Design review of the part built by this model. Coordinates are the model's own, in mm. Face numbers are marked on the shaded views. A direction names the side the tool comes from. Round coordinates to 2 decimals unless told otherwise and drop trailing zeros. Write each loop counter-clockwise with the first axis right and the second up, starting at its lowest first coordinate (ties: lowest second). Pieces come first, ordered by that corner, then holes.
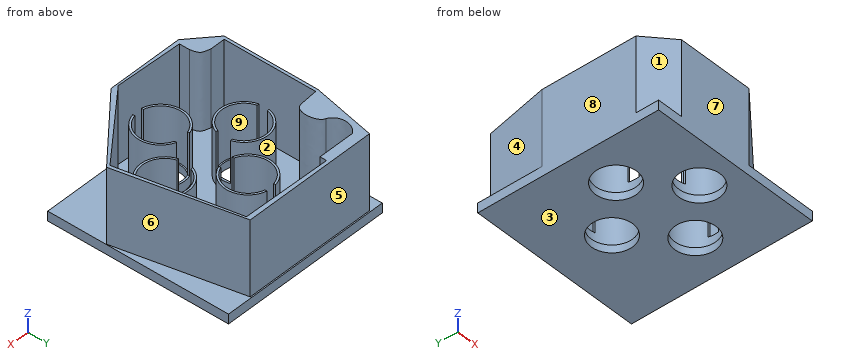
from build123d import *

# Parameters (mm, degrees)
F1_DEPTH  = 220
F3_W      = 450
F3_H      = 470
F4_DEPTH  = 25
F5_DEPTH  = 200
F6_R      = 53.5
F7_DEPTH  = 20
F6_R_2    = 62
F6_R_3    = 57
F8_DEPTH  = 154
F9_W      = 25.5
F9_H      = 90.3576454148
F9_W_2    = 90.3576454148
F9_H_2    = 25.5
F10_DEPTH = 175


with BuildPart() as f1:
    # F0 (on Top) → F1 (new body)
    with BuildSketch(Plane.XY):
        Polygon((-204.7800719738, 171.1511015892), (-238.562181592, 7.3397289511), (-238.562181592, -236.6909831762), (-171.305090189, -295.6561148167), (26.1666476727, -295.6561148167), (210.4326635599, -143.6366438866), (144.4040089846, 171.1511015892), align=None)
    extrude(amount=F1_DEPTH)

    # F3 (on Top) → F4 (join)
    with BuildSketch(Plane.XY):
        with Locations((-13.562181592, -60.6561148167)):
            Rectangle(F3_W, F3_H)
    extrude(amount=F4_DEPTH)

    # F2 (on face) → F5 (cut)
    with BuildSketch(Plane.XY.offset(220)):
        with BuildLine():
            Line((141.9471204281, 159.1738164425), (-88.6924937367, 162.5520288944))
            Line((-88.6924937367, 162.5520288944), (-88.6924937367, 145.6609666348))
            Line((-88.6924937367, 145.6609666348), (-182.9752624035, 145.6609666348))
            add(Edge.make_bspline(
                [(-182.9752624035, 145.6609666348), (-207.5440585613, 131.841018796), (-210.6151580811, 91.9167175889), (-182.9752624035, 77.1754458547)],
                knots=[0, 0, 0, 0, 68.4855207801, 68.4855207801, 68.4855207801, 68.4855207801], degree=3))
            add(Edge.make_bspline(
                [(-182.9752624035, 77.1754458547), (-164.8557782173, 75.025677681), (-155.0282537937, 17.2889921814), (-182.9752624035, 12.0681189001)],
                knots=[0, 0, 0, 0, 65.1073269546, 65.1073269546, 65.1073269546, 65.1073269546], degree=3))
            Line((-182.9752624035, 12.0681189001), (-231.1915457249, 7.7685844153))
            Line((-231.1915457249, 7.7685844153), (-231.1915457249, -229.9345582724))
            Line((-231.1915457249, -229.9345582724), (-191.8814480305, -229.9345582724))
            add(Edge.make_bspline(
                [(-191.8814480305, -229.9345582724), (-168.2339906693, -236.6909831762), (-168.2339906693, -236.6909831762), (-163.0131155252, -259.417116642)],
                knots=[0, 0, 0, 0, 41.2625964967, 41.2625964967, 41.2625964967, 41.2625964967], degree=3))
            Line((-163.0131155252, -259.417116642), (-163.0131155252, -285.8285903931))
            Line((-163.0131155252, -285.8285903931), (10.1969307289, -291.0494506359))
            Line((10.1969307289, -291.0494506359), (201.833575964, -142.4082070589))
            Line((201.833575964, -142.4082070589), (141.9471204281, 159.1738164425))
        make_face()
    extrude(amount=-F5_DEPTH, mode=Mode.SUBTRACT)

    # F6 (on Top) → F7 (cut, through all)
    with BuildSketch(Plane.XY):
        with Locations((-14.6330455318, 24.2691934109)):
            Circle(F6_R)
        with Locations((-128.4027075395, -87.3125935497)):
            Circle(F6_R)
        with Locations((-14.7721923306, -203.1711548904)):
            Circle(F6_R)
        with Locations((98.9974696771, -91.5893679298)):
            Circle(F6_R)
    extrude(amount=F7_DEPTH, mode=Mode.SUBTRACT)

    # F6 (on Top) → F8 (join)
    with BuildSketch(Plane.XY):
        with Locations((98.9974696771, -91.5893679298)):
            Circle(F6_R_2)
        with Locations((98.9974696771, -91.5893679298)):
            Circle(F6_R_3, mode=Mode.SUBTRACT)
        with Locations((-14.6330455318, 24.2691934109)):
            Circle(F6_R_2)
        with Locations((-14.6330455318, 24.2691934109)):
            Circle(F6_R_3, mode=Mode.SUBTRACT)
        with Locations((-128.4027075395, -87.3125935497)):
            Circle(F6_R_2)
        with Locations((-128.4027075395, -87.3125935497)):
            Circle(F6_R_3, mode=Mode.SUBTRACT)
        with Locations((-14.7721923306, -203.1711548904)):
            Circle(F6_R_2)
        with Locations((-14.7721923306, -203.1711548904)):
            Circle(F6_R_3, mode=Mode.SUBTRACT)
    extrude(amount=F8_DEPTH)

    # F9 (on face) → F10 (cut)
    with BuildSketch(Plane.XY.offset(220)):
        Polygon((-14.3728665248, -89.0469396694), (4.8721171106, -89.0469396694), (4.8821498398, -89.0469396694), (4.8821498398, -69.801956034), (-14.3728665248, -69.801956034), align=None)
        Polygon((4.8721171106, -108.301956034), (4.8721171106, -89.0469396694), (-14.3728665248, -89.0469396694), (-14.3728665248, -108.2919233048), (-14.3728665248, -108.301956034), align=None)
        Polygon((4.8821498398, -89.0469396694), (4.8721171106, -89.0469396694), (4.8721171106, -108.301956034), (89.2823901994, -108.301956034), (89.2823901994, -101.801956034), (89.2823901994, -76.301956034), (89.2823901994, -69.801956034), (4.8821498398, -69.801956034), align=None)
        Polygon((-14.3728665248, -108.2919233048), (-14.3728665248, -89.0469396694), (-33.6178501602, -89.0469396694), (-33.6278828894, -89.0469396694), (-33.6278828894, -108.2919233048), align=None)
        Polygon((-33.6178501602, -89.0469396694), (-14.3728665248, -89.0469396694), (-14.3728665248, -69.801956034), (-14.3728665248, -69.7919233048), (-33.6178501602, -69.7919233048), align=None)
        Polygon((4.8721171106, -192.7021963936), (4.8721171106, -108.301956034), (-14.3728665248, -108.301956034), (-14.3728665248, -108.2919233048), (-33.6278828894, -108.2919233048), (-33.6278828894, -192.7021963936), (-27.1278828894, -192.7021963936), (-1.6278828894, -192.7021963936), align=None)
        Polygon((-14.3728665248, -69.801956034), (4.8821498398, -69.801956034), (4.8821498398, 14.6083170548), (-1.6178501602, 14.6083170548), (-27.1178501602, 14.6083170548), (-33.6178501602, 14.6083170548), (-33.6178501602, -69.7919233048), (-14.3728665248, -69.7919233048), align=None)
        Polygon((-33.6278828894, -89.0469396694), (-33.6178501602, -89.0469396694), (-33.6178501602, -69.7919233048), (-118.028123249, -69.7919233048), (-118.028123249, -76.2919233048), (-118.028123249, -101.7919233048), (-118.028123249, -108.2919233048), (-33.6278828894, -108.2919233048), align=None)
        with Locations((-14.3778828894, -237.881019101)):
            Rectangle(F9_W, F9_H)
        with Locations((134.4612129068, -89.051956034)):
            Rectangle(F9_W_2, F9_H_2)
        with Locations((-14.3678501602, 59.7871397622)):
            Rectangle(F9_W, F9_H)
        with Locations((-163.2069459564, -89.0419233048)):
            Rectangle(F9_W_2, F9_H_2)
    extrude(amount=-F10_DEPTH, mode=Mode.SUBTRACT)


solid = f1.part
1) For line 1 along X through (y, z) = (-125.5, 57.5); line 2 along X through (y, z) = (30.5, 88.5); line 3 along Y through (x, z) = (-60, 138), list the stretches that pass through material, from the lowest coordinate up.
2) The part is to be moulded in two halves that separate along X. For the marked faces 6, 7, 8 and 9, say which applies: pulls with the +X half, pulls with the -X half, needs draft (parallel to the pull), parting line crosses it, or undercut.
3) Add section A-A on x = -10. Count the separate pieces of the cut face and the enclosed holes in it, and give its area (3 significant figures).
4) For P1, Ø4, axis at x = -9.5, y = -144, coming from the +Z side; P2, Ø2.5, axis at x = 41.5, z = 89, coming from the +Y side; P3, Ø4, axis at x = 76.5, z = 97.5, coming from the -Y side; P4, Ø6, axis at y = -163, z = 26, coming from the +X side, all flat-tipped, find the tip position at first contact; note any pin that passes through.
5) For the marked faces 1, 2, 3, 4 and 5, list the 3-axis set-ups (+Z, -Z, +X, -X, +Y, -Y) from which the entire face can be reached by the end or side of a thin tool; tool diameter is ignored.
6) Add section D-D on y = -10.5. State the section outline as (x, z) points, and give its area (3 significant figures).
7) Add section C-C on x = 110.5. State the section outline as (y, z) points, and give its area (3 significant figures).
Computed:
1. line 1: x = -238.56 to -231.19, -177.25 to -170.72, -86.09 to -79.56, 47.09 to 53.18, 144.81 to 150.9, 198.48 to 206.63
1. line 2: x = -233.79 to -166.59, -76.32 to -71.29, 42.03 to 47.05, 167.5 to 173.91
1. line 3: y = -295.66 to -288.93, -245.58 to -237.86, -168.48 to -160.76, -17.99 to -10.24, 58.78 to 66.53, 162.13 to 171.15
2. face 6: pulls with the +X half
2. face 7: needs draft
2. face 8: pulls with the -X half
2. face 9: undercut
3. separate pieces: 3
3. enclosed holes: 0
3. area: 8,650 mm2
4. P1: stops at z = 45
4. P2: stops at y = 171.15
4. P3: stops at y = -255.78
4. P4: stops at x = 211.44
5. face 1: +Z, -X, -Y
5. face 2: +Z
5. face 3: -Z, +X, -X, +Y, -Y
5. face 4: +Z, -X, +Y
5. face 5: +Z, +X, -X, +Y
6. outline: (-238.56, 0) - (-55.29, 0) - (-55.29, 20) - (-59.8, 20) - (-59.8, 154) - (-65.97, 154) - (-65.97, 20) - (-231.19, 20) - (-231.19, 220) - (-238.56, 220) - close; (26.03, 0) - (211.44, 0) - (211.44, 25) - (182.51, 25) - (182.51, 220) - (175.64, 220) - (175.64, 20) - (36.7, 20) - (36.7, 154) - (30.53, 154) - (30.53, 20) - (26.03, 20) - close
6. area: 12,000 mm2
7. outline: (-295.66, 0) - (-143.84, 0) - (-143.84, 20) - (-147.42, 20) - (-147.42, 154) - (-152.51, 154) - (-152.51, 20) - (-213.25, 20) - (-213.25, 220) - (-226.08, 220) - (-226.08, 25) - (-295.66, 25) - close; (-39.34, 0) - (174.34, 0) - (174.34, 25) - (171.15, 25) - (171.15, 220) - (159.63, 220) - (159.63, 20) - (-30.67, 20) - (-30.67, 154) - (-35.76, 154) - (-35.76, 20) - (-39.34, 20) - close
7. area: 13,900 mm2
